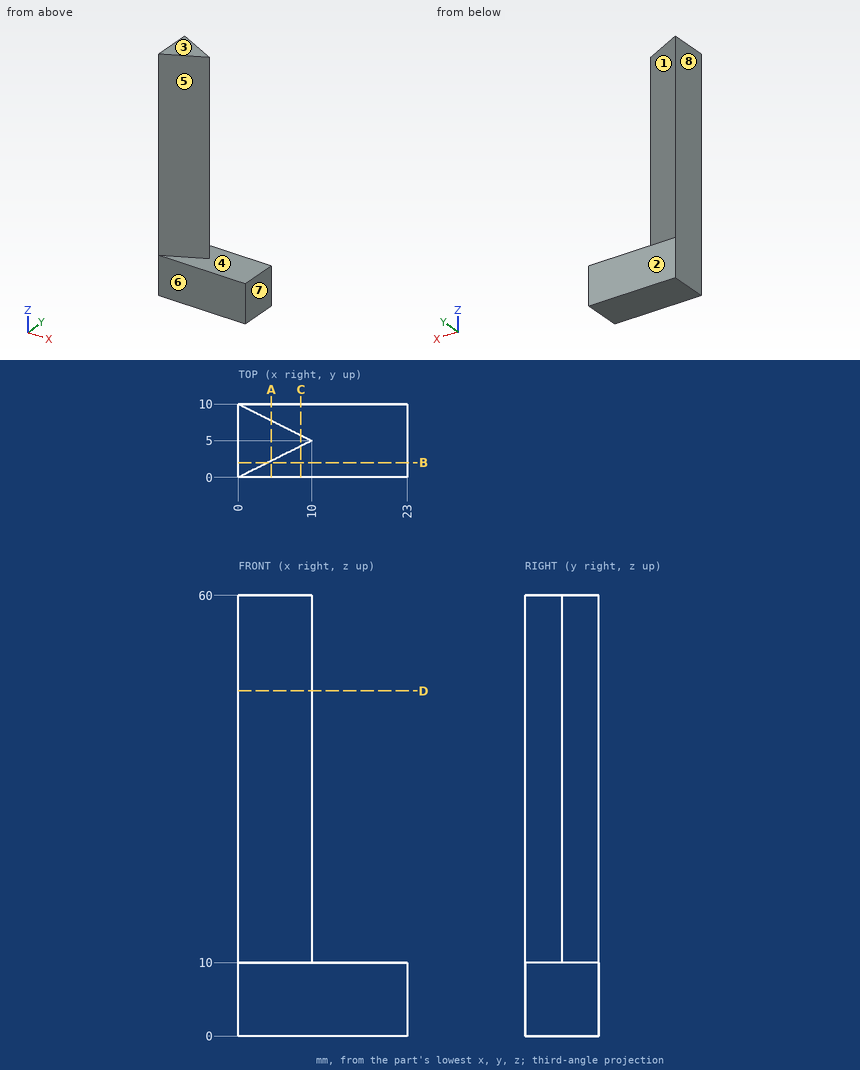
Geometry: see drawing. Coordinates: mm, zero at the bounding-box minimum. A direction names the side the tool comes from. Give positions to 0.01 mm unless a question says otherwise; leave off trailing zeros. Order: outer loops, then holes, each group sorted by start corner. A loop starts at its lowest first (then second) coordinate and runs counter-clockwise, first axis right, second up. Notation, with made-up numbers: (-15, 47) - (19, 47) arc R23 cw to (19, 75) - close; hole circle Ø7 at (15, 5). An arc over 180 degrees is marked (long way). Write each question's results on one line, items separated by ' | '.
Item 1: Section C-C (x = 8.5). Return loops of the section in (y, z).
A:
outline: (0, 0) - (10, 0) - (10, 10) - (5.75, 10) - (5.75, 60) - (4.25, 60) - (4.25, 10) - (0, 10) - close
Item 2: Section D-D (z = 47). Return loops of the section in (x, y).
A:
outline: (0, 0) - (10, 5) - (0, 10) - close
Item 3: Section A-A (x = 4.5). Return loops of the section in (y, z), and give its area (3 significant figures).
A:
outline: (0, 0) - (10, 0) - (10, 10) - (7.75, 10) - (7.75, 60) - (2.25, 60) - (2.25, 10) - (0, 10) - close | area: 375 mm^2
Item 4: Section B-B (y = 2). Return loops of the section in (x, z).
A:
outline: (0, 0) - (23, 0) - (23, 10) - (4, 10) - (4, 60) - (0, 60) - close
Item 5: Access query for the marked faces 1, 2, 3, 4 and 5. Directions: +Z, -Z, +X, -X, +Y, -Y. A direction counts if a zero-diameter tool reaches every point of the face in a straight line with its end or side. Return the directions, or none.
A:
face 1: +Z, +X, +Y | face 2: +Z, -Z, +X, -X, +Y | face 3: +Z, +X, -X, +Y, -Y | face 4: +Z, +X | face 5: +Z, +X, -Y
Item 6: Contact query for flat-ended pins moving along their axis: pin 1 Ø4 at (x, y) = (18, 2.5) entering from +Z; pin 2 Ø4 at (x, z) = (6, 43) entering from +Y. Output: stop coordinate, or through.
A:
pin 1: stops at z = 10 | pin 2: stops at y = 8
Item 7: Material intervals for line 1 along Z through (x, y) = (18.5, 1.25); line 2 along X through (y, z) = (8.5, 15); line 3 along X through (y, z) = (7, 19.5), sorted ascending.
A:
line 1: z = 0 to 10 | line 2: x = 0 to 3 | line 3: x = 0 to 6
Item 8: Draft query along X for the marked faces 6, 7 and 8. Return one class per face: released by +X, released by -X, zero draft, split by the parting line, or undercut.
A:
face 6: zero draft | face 7: released by +X | face 8: released by -X
